Geometry: final body of the model. Coordinates: model frame, mm. Face numbers are marked on the shaded views. A direction names the side the tool comes from. Give positions to 0.01 mm unless a question says otherwise; leave off trailing zeros. Write each loop counter-clockwise with the first axis right and the second up, starting at its lowest first coordinate (ties: lowest second). Pieces come first, ordered by that corner, then holes. Notation, with made-up numbers: M 9.5,-17 L 55.5,-17 A18 cw 55.5,-3 Z; hole C -11,11.25 d4. An arc over 180 degrees is marked long. Use a Markdown table: item, result. Add a question column.
(1) Cut plane A-A (x = 21). Output: boundary loops of the cut face in (y, z).
(2) Reachability of the marked faces 1 and 2 from +Z, -Z, +X, -X, +Y, -Y: full face, straight path, thin tool, end or side. Return the list, or none.
(3) Cut plane C-C (y = 0). Output: boundary loops of the cut face in (x, z).
(4) Material intervals for L1, parallel to Y at x = 21, z = 0.2; L2, parallel to Z at x = -21.15, y = -10; L3, parallel to Z at x = 14.5, y = 7.5, sorted ascending.
(5) Pin query (flat end, axial travel): pin 1 Ø1.6 at (x, z) = (-21.5, -1.5) entering from -Y; pin 2 Ø2.5 at (y, z) = (10, -3.5) entering from -X; pin 3 Ø1 at (x, z) = (-22, -3) entering from +Y; pin 4 Ø13.5 at (x, y) = (-8.5, -8.5) entering from -Z. Return the tip coordinate at first contact, or that it passes through.
(6) Cut plane B-B (y = 21). Output: boundary loops of the cut face in (x, z).
(7) Cut plane D-D (x = 8). Output: boundary loops of the cut face in (y, z), plus the area to 3 significant figures.
```python
from build123d import *

# Parameters (mm, degrees)
EXTRUDE_1_DEPTH     = 1
SKETCH_2_W          = 2
SKETCH_2_H          = 29
EXTRUDE_2_DEPTH     = 7
SKETCH_3_R          = 1.1
CUT_EXTRUDE_1_DEPTH = 7
SKETCH_4_R          = 0.8
CUT_EXTRUDE_2_DEPTH = 7
CHAMFER_1_SIZE      = 0.5
FILLET_1_R          = 4
CUT_EXTRUDE_3_DEPTH = 10


with BuildPart() as part:
    # 草图1 → 凸台-拉伸1 (new body)
    with BuildSketch(Plane.XY):
        with BuildLine():
            Line((22.5, -21.8), (22.5, 21.8))
            ThreePointArc((22.5, 21.8), (22.294974747, 22.294974747), (21.8, 22.5))
            Line((21.8, 22.5), (-21.8, 22.5))
            ThreePointArc((-21.8, 22.5), (-22.294974747, 22.294974747), (-22.5, 21.8))
            Line((-22.5, 21.8), (-22.5, -21.8))
            ThreePointArc((-22.5, -21.8), (-22.294974747, -22.294974747), (-21.8, -22.5))
            Line((-21.8, -22.5), (21.8, -22.5))
            ThreePointArc((21.8, -22.5), (22.294974747, -22.294974747), (22.5, -21.8))
        make_face()
    extrude(amount=EXTRUDE_1_DEPTH)

    # 草图2 → 凸台-拉伸2 (add)
    with BuildSketch(Plane(origin=(0, 0, 0), x_dir=(-1, 0, 0), z_dir=(0, 0, -1))):
        with Locations((21.5, 0)):
            Rectangle(SKETCH_2_W, SKETCH_2_H)
    extrude(amount=EXTRUDE_2_DEPTH)

    # 草图3 → 切除-拉伸1 (cut)
    with BuildSketch(Plane(origin=(0, 0, 0), x_dir=(-1, 0, 0), z_dir=(0, 0, -1))):
        with Locations((-21, 21)):
            Circle(SKETCH_3_R)
        with Locations((-21, -21)):
            Circle(SKETCH_3_R)
    extrude(amount=-CUT_EXTRUDE_1_DEPTH, mode=Mode.SUBTRACT)

    # 草图4 → 切除-拉伸2 (cut)
    with BuildSketch(Plane.ZY.offset(22.5)):
        with Locations(Location((-3.5, 10, 0), (0, 0, 270))):
            Circle(SKETCH_4_R)
        with Locations(Location((-3.5, -10, 0), (0, 0, 270))):
            Circle(SKETCH_4_R)
    extrude(amount=-CUT_EXTRUDE_2_DEPTH, mode=Mode.SUBTRACT)

    # 倒角1
    # the kernel refuses this chamfer: 0.5 mm, written as the material it takes off along each edge
    with BuildSketch(Plane(origin=(21, 21, 1), x_dir=(-1, 0, 0), z_dir=(0, -1, 0))) as chamfer_1_piece_1:
        Polygon((1.1 + CHAMFER_1_SIZE, 0), (1.1, CHAMFER_1_SIZE), (1.1, 0), align=None)
    revolve(axis=Axis((21, 21, 1), (0, 0, -1)), mode=Mode.SUBTRACT)
    with BuildSketch(Plane(origin=(21, -21, 1), x_dir=(-1, 0, 0), z_dir=(0, -1, 0))) as chamfer_1_piece_2:
        Polygon((1.1 + CHAMFER_1_SIZE, 0), (1.1, CHAMFER_1_SIZE), (1.1, 0), align=None)
    revolve(axis=Axis((21, -21, 1), (0, 0, -1)), mode=Mode.SUBTRACT)

    # 圆角1
    fillet_1_edges = [part.edges().sort_by_distance(p)[0] for p in [
        (-21.5, 14.5, -7),
        (-21.5, -14.5, -7),
    ]]
    fillet(fillet_1_edges, radius=FILLET_1_R)

    # 草图5 → 切除-拉伸3 (cut)
    with BuildSketch(Plane.ZY.offset(22.5)):
        with BuildLine():
            Line((-4.5, 5), (-1.5, 5))
            ThreePointArc((-1.5, 5), (-0.792893219, 4.707106781), (-0.5, 4))
            Line((-0.5, 4), (-0.5, -4))
            ThreePointArc((-0.5, -4), (-0.792893219, -4.707106781), (-1.5, -5))
            Line((-1.5, -5), (-4.5, -5))
            ThreePointArc((-4.5, -5), (-5.207106781, -4.707106781), (-5.5, -4))
            Line((-5.5, -4), (-5.5, 4))
            ThreePointArc((-5.5, 4), (-5.207106781, 4.707106781), (-4.5, 5))
        make_face()
    extrude(amount=-CUT_EXTRUDE_3_DEPTH, mode=Mode.SUBTRACT)


solid = part.part
```
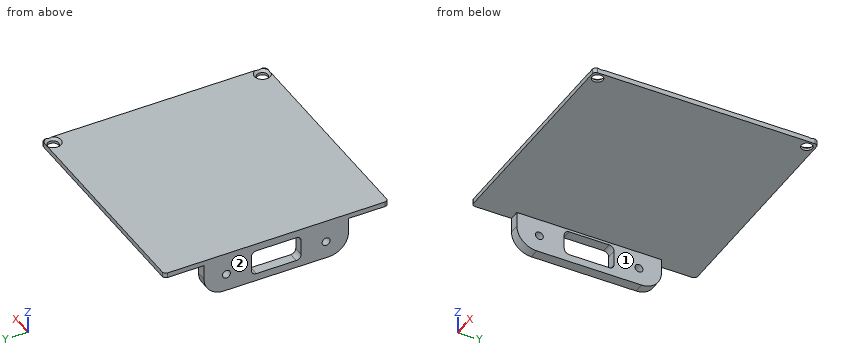
Answer list:
| question | item | result |
|---|---|---|
| 1 | outline | M -22.5,0 L -22.1,0 L -22.1,0.5 L -22.5,0.9 Z; M -19.9,0 L 19.9,0 L 19.9,0.5 L 19.4,1 L -19.4,1 L -19.9,0.5 Z; M 22.1,0 L 22.5,0 L 22.5,0.9 L 22.1,0.5 Z |
| 2 | face 1 | -Z, +X, +Y, -Y |
| 2 | face 2 | +Z, -Z, -X, +Y, -Y |
| 3 | outline | M -22.5,-7 L -20.5,-7 L -20.5,-5.5 L -22.5,-5.5 Z; M -22.5,-0.5 L -20.5,-0.5 L -20.5,0 L 22.5,0 L 22.5,1 L -22.5,1 Z |
| 4 | L1 | -22.5 to -22.1, -19.9 to 19.9, 22.1 to 22.5 |
| 4 | L2 | -7 to -4.3, -2.7 to 1 |
| 4 | L3 | 0 to 1 |
| 5 | pin 1 | y = -14.5 |
| 5 | pin 2 | x = -22.5 |
| 5 | pin 3 | y = 14.5 |
| 5 | pin 4 | z = 0 |
| 6 | outline | M -22.5,0 L 19.9,0 L 19.9,0.5 L 19.4,1 L -22.5,1 Z; M 22.1,0 L 22.5,0 L 22.5,0.9 L 22.1,0.5 Z |
| 7 | outline | M -22.5,0 L 22.5,0 L 22.5,1 L -22.5,1 Z |
| 7 | area | 45.0 mm² |
